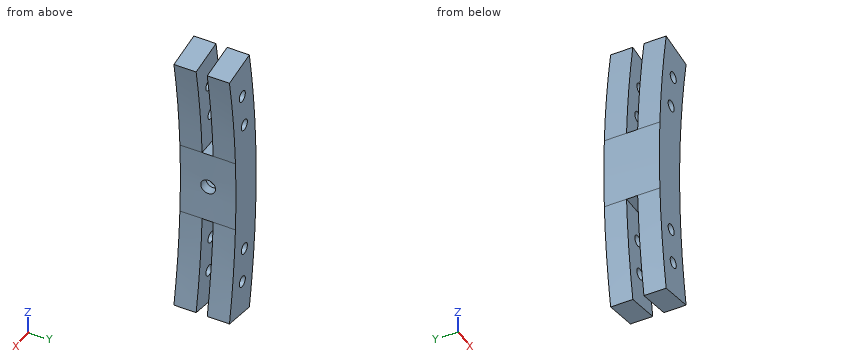
from build123d import *

# Parameters (mm, degrees)
BASE2_DEPTH            = 7.5
MOUNT2_START           = -1.5
MOUNT2_DEPTH           = 3
MOUNT_HOLE2_DEPTH      = 224.418192135
MOUNT_HOLE2_DEPTH_BACK = 224.418192135
SKETCH16_R             = 1.5
SKETCH17_R             = 2
SHAFT_HOLE_DEPTH       = 40.784051683
SKETCH18_W             = 2.5
SKETCH18_H             = 3.5


with BuildPart() as part:
    # Sketch13 → base2 (new, symmetric)
    with BuildSketch(Plane(origin=(0, 0, 0), x_dir=(1, 0, 0), z_dir=(0, 1, 0))):
        with BuildLine():
            ThreePointArc((-209.761769634, 10), (-208.70564487, 23.279901188), (-206.809628133, 36.46611731))
            Line((-206.809628133, 36.46611731), (-216.657705663, 38.202599087))
            ThreePointArc((-216.657705663, 38.202599087), (-218.670303662, 24.151569236), (-219.772609758, 10))
            Line((-219.772609758, 10), (-209.761769634, 10))
        make_face()
        with BuildLine():
            ThreePointArc((-209.761769634, -10), (-210, 0), (-209.761769634, 10))
            Line((-209.761769634, 10), (-219.772609758, 10))
            ThreePointArc((-219.772609758, 10), (-220, 0), (-219.772609758, -10))
            Line((-219.772609758, -10), (-209.761769634, -10))
        make_face()
        with BuildLine():
            Line((-216.657705663, -38.202599087), (-206.809628133, -36.46611731))
            ThreePointArc((-206.809628133, -36.46611731), (-208.70564487, -23.279901188), (-209.761769634, -10))
            Line((-209.761769634, -10), (-219.772609758, -10))
            ThreePointArc((-219.772609758, -10), (-218.670303662, -24.151569236), (-216.657705663, -38.202599087))
        make_face()
    extrude(amount=BASE2_DEPTH, both=True)

    # Sketch14 → mount2 (cut)
    with BuildSketch(Plane(origin=(0, 0, 0), x_dir=(1, 0, 0), z_dir=(0, 1, 0)).offset(MOUNT2_START)):
        with BuildLine():
            Line((-209.761769634, -10), (-219.772609758, -10))
            ThreePointArc((-219.772609758, -10), (-218.670303662, -24.151569236), (-216.657705663, -38.202599087))
            Line((-216.657705663, -38.202599087), (-206.809628133, -36.46611731))
            ThreePointArc((-206.809628133, -36.46611731), (-208.70564487, -23.279901188), (-209.761769634, -10))
        make_face()
        with BuildLine():
            Line((-209.761769634, 10), (-219.772609758, 10))
            ThreePointArc((-219.772609758, 10), (-218.670303662, 24.151569236), (-216.657705663, 38.202599087))
            Line((-216.657705663, 38.202599087), (-206.809628133, 36.46611731))
            ThreePointArc((-206.809628133, 36.46611731), (-208.70564487, 23.279901188), (-209.761769634, 10))
        make_face()
    extrude(amount=MOUNT2_DEPTH, mode=Mode.SUBTRACT)

    # Sketch16 → mount hole2 (cut, two sides: drawn at the far end of the back side and taken through both)
    with BuildSketch(Plane(origin=(0, 0, 0), x_dir=(1, 0, 0), z_dir=(0, 1, 0)).offset(-MOUNT_HOLE2_DEPTH_BACK)):
        with Locations(Location((-213.160645195, 28.063131327, 0), (0, 0, 270))):
            Circle(SKETCH16_R)
        with Locations(Location((-214.18186009, 18.738484691, 0), (0, 0, 270))):
            Circle(SKETCH16_R)
        with Locations(Location((-214.18186009, -18.738484691, 0), (0, 0, 270))):
            Circle(SKETCH16_R)
        with Locations(Location((-213.160645195, -28.063131327, 0), (0, 0, 270))):
            Circle(SKETCH16_R)
    extrude(amount=MOUNT_HOLE2_DEPTH + MOUNT_HOLE2_DEPTH_BACK, mode=Mode.SUBTRACT)

    # Sketch17 → shaft hole (cut, through all)
    with BuildSketch(Plane(origin=(-215, 0, 0), x_dir=(0, 0, -1), z_dir=(1, 0, 0))):
        with Locations(Location((0, 0, 0), (0, 0, 180))):
            Circle(SKETCH17_R)
    extrude(amount=SHAFT_HOLE_DEPTH, mode=Mode.SUBTRACT)

    # Sketch18 → bearinghole (revolve, cut)
    with BuildSketch(Plane(origin=(0, 0, 0), x_dir=(1, 0, 0), z_dir=(0, 1, 0)), mode=Mode.PRIVATE) as bearinghole_sk:
        with Locations((-213.75, 1.75)):
            Rectangle(SKETCH18_W, SKETCH18_H)
    revolve(bearinghole_sk.sketch.rotate(Axis((-215, 0, 0), (1, 0, 0)), 180), axis=Axis((-215, 0, 0), (1, 0, 0)), mode=Mode.SUBTRACT)


solid = part.part
Can you work these out from the model? Positions are in its coordinate system, mm. Coordinates: 2 decimals unless noted, no trailing zeros. Write each loop counter-clockwise with the first axis right and the second up, starting at its lowest first coordinate (ties: lowest second). Pieces come first, ordered by that corner, then holes. Notation, with made-up numbers: (18.25, -3.75) - (28.25, -3.75) arc R13 cw to (28.25, 4.25) - close; hole circle Ø1 at (-10, 65.5). An arc over 180 degrees is marked (long way). Return JSON: item names as keys, results as strings. Group by question number.
Item 1: If we section it at D-D (x = -208.5): Write out the boundary of the cut face in (y, z), then the cut area to 3 significant figures.
Item 2: If we section it at A-A (y = 0): Write out the boundary of the cut face in (x, z).
Item 3: Please list where these lines run through material, in increasing order: probe 1 along Y at (x, z) = (-214.75, -22.5); probe 2 along Z at (x, y) = (-214.5, 4.75); probe 3 along Z at (x, y) = (-213.5, -6).
Item 4: I'm going to push flat-ended pins straight in: pin 1 Ø6 at (y, z) = (-4.5, 10) entering from -X; pin 2 Ø3 at (y, z) = (3.5, 4) entering from +X; pin 3 Ø1 at (x, z) = (-209, -13.5) entering from +Y; pin 4 Ø2.5 at (x, y) = (-213, 0.5) entering from -Z. Where does each tip first touch, or does it pass through?
Item 5: If we section it at B-B (z = -28.5): Write out the boundary of the cut face in (x, y), then the cut area to 3 significant figures.
Item 6: If we section it at C-C (z = -11): Write out the boundary of the cut face in (x, y).
Return value:
{
 "1": {"outline": "(-7.5, -36.76) - (-1.5, -36.76) - (-1.5, -25.05) - (-7.5, -25.05) - close; (-7.5, 25.05) - (-1.5, 25.05) - (-1.5, 36.76) - (-7.5, 36.76) - close; (1.5, -36.76) - (7.5, -36.76) - (7.5, -25.05) - (1.5, -25.05) - close; (1.5, 25.05) - (7.5, 25.05) - (7.5, 36.76) - (1.5, 36.76) - close", "area": "281 mm^2"},
 "2": {"outline": "(-219.77, -10) - (-209.76, -10) arc R210 cw to (-209.99, -2) - (-212.5, -2) - (-212.5, -3.5) - (-215, -3.5) - (-215, 3.5) - (-212.5, 3.5) - (-212.5, 2) - (-209.99, 2) arc R210 cw to (-209.76, 10) - (-219.77, 10) arc R220 ccw to start"},
 "3": {"probe 1": "y = -7.5 to -1.5, 1.5 to 7.5", "probe 2": "z = -37.82 to -28.74, -27.39 to -20.2, -17.27 to 17.27, 20.2 to 27.39, 28.74 to 37.82", "probe 3": "z = -37.65 to -29.52, -26.6 to -20.07, -17.4 to 17.4, 20.07 to 26.6, 29.52 to 37.65"},
 "4": {"pin 1": "stops at x = -219.89", "pin 2": "stops at x = -209.93", "pin 3": "passes through", "pin 4": "stops at z = -37.69"},
 "5": {"outline": "(-218.15, -7.5) - (-214.6, -7.5) - (-214.6, -1.5) - (-218.15, -1.5) - close; (-218.15, 1.5) - (-214.6, 1.5) - (-214.6, 7.5) - (-218.15, 7.5) - close; (-211.73, -7.5) - (-208.06, -7.5) - (-208.06, -1.5) - (-211.73, -1.5) - close; (-211.73, 1.5) - (-208.06, 1.5) - (-208.06, 7.5) - (-211.73, 7.5) - close", "area": "86.6 mm^2"},
 "6": {"outline": "(-219.72, -7.5) - (-209.71, -7.5) - (-209.71, -1.5) - (-219.72, -1.5) - close; (-219.72, 1.5) - (-209.71, 1.5) - (-209.71, 7.5) - (-219.72, 7.5) - close"}
}
